from build123d import *

# Parameters (mm, degrees)
F0_W     = 122
F0_H     = 44
F0_R     = 2
F1_DEPTH = 1.6
F2_W     = 106
F2_H     = 35
F3_DEPTH = 8.5
F5_DEPTH = 3.5


with BuildPart() as f1:
    # F0 (on Front) → F1 (new body)
    with BuildSketch(Plane.XZ):
        Rectangle(F0_W, F0_H)
        with Locations((-57.5, -18.5)):
            Circle(F0_R, mode=Mode.SUBTRACT)
        with Locations((57.5, -18.5)):
            Circle(F0_R, mode=Mode.SUBTRACT)
        with Locations((-57.5, 18.5)):
            Circle(F0_R, mode=Mode.SUBTRACT)
        with Locations((57.5, 18.5)):
            Circle(F0_R, mode=Mode.SUBTRACT)
    extrude(amount=-F1_DEPTH)

    # F2 (on Front) → F3 (join)
    with BuildSketch(Plane.XZ):
        with Locations((0, 2.25)):
            Rectangle(F2_W, F2_H)
    extrude(amount=F3_DEPTH)

    # F4 (on Front) → F5 (join)
    with BuildSketch(Plane.XZ):
        Polygon((53, 15.300509), (53, -13.699491), (57.8, -8.899491), (57.8, 10.500509), align=None)
    extrude(amount=F5_DEPTH)


solid = f1.part
Geometry check sheet. Reference: the model listing, model coordinates, mm. A direction names the side the tool comes from. Round coordinates to 2 decimals unless told otherwise and drop trailing zeros. Order: outer loops, then holes, each group sorted by start corner. A loop starts at its lowest first (then second) coordinate and runs counter-clockwise, first axis right, second up. Notation, with made-up numbers: (16.5, 43) - (25.5, 43) arc R23 ccw to (25.5, 53) - close; hole circle Ø9 at (8, 19). An arc over 180 degrees is marked (long way). One line per question, with ' | ' between items. Start each with the question number.
(1) Sectioned sample at C-C on x = -57.5. Record the cut outline in (y, z).
(2) Access from +Z, -Z, +X, -X, +Y, -Y to the whole of each face (thin tool, end or side, straight path). Record for faces 1 (the flat face through (-53, -4, 2)), 2 (the flat face through (55.4, -1.7, 12.9)), 3 (the flat face through (57.8, -2, 1)), 4 (the flat face through (-1, -4, 19.75)), 5 (the flat face through (-1, -4, -15.25)).
(3) Thickness scan on L1, parallel to Z at x = -57.5, y = 0.3; L2, parallel to X at y = -0.5, z = 19; L3, parallel to Z at x = 11.5, y = -1. Record the ranges inside material, lowest first. Write a range as [from, to].
(4) Sectioned sample at D-D on x = -41. Record the cut outline in (y, z).
(5) Release check for a two-part mould opening along Z. For faces 6 (the flat face through (53, -6, 2)), 7 (the flat face through (55.4, -1.7, -11.3)), 8 (the cylindrical face through (59.408, 0.789, 19.101)) record: released by +Z, released by -Z, zero draft, split by the parting line, or undercut.
(6) Depth check by flat-ended pin: pin 1 Ø3 at (y, z) = (-2, 1.5) entering from +X; pin 2 Ø4 at (x, y) = (-33.5, -6.5) entering from +Z; pin 3 Ø1.5 at (x, y) = (-20.5, -5) entering from -Z. Enter the tip coordinate at first touch or a pass-through.
(7) Sectioned sample at B-B on y = -2. Record the cut outline in (x, z), and give its area (3 significant figures).
(8) Sectioned sample at A-A on z = -18.5. Record the cut outline in (x, y).
Conclusion:
1) outline: (0, -22) - (1.6, -22) - (1.6, -20.5) - (0, -20.5) - close; (0, -16.5) - (1.6, -16.5) - (1.6, 16.5) - (0, 16.5) - close; (0, 20.5) - (1.6, 20.5) - (1.6, 22) - (0, 22) - close
2) face 1: +Z, -Z, -X, -Y | face 2: +Z, +X, -Y | face 3: +Z, -Z, +X, -Y | face 4: +Z, +X, -X, -Y | face 5: -Z, +X, -X, -Y
3) L1: z = [-22, -20.5], [-16.5, 16.5], [20.5, 22] | L2: x = [-53, 53] | L3: z = [-15.25, 19.75]
4) outline: (-8.5, -15.25) - (0, -15.25) - (0, -22) - (1.6, -22) - (1.6, 22) - (0, 22) - (0, 19.75) - (-8.5, 19.75) - close
5) face 6: zero draft | face 7: released by -Z | face 8: undercut
6) pin 1: stops at x = 57.8 | pin 2: stops at z = 19.75 | pin 3: stops at z = -15.25
7) outline: (-53, -15.25) - (53, -15.25) - (53, -13.7) - (57.8, -8.9) - (57.8, 10.5) - (53, 15.3) - (53, 19.75) - (-53, 19.75) - close | area: 3,830 mm2
8) outline: (-61, 0) - (-59.5, 0) - (-59.5, 1.6) - (-61, 1.6) - close; (-55.5, 0) - (55.5, 0) - (55.5, 1.6) - (-55.5, 1.6) - close; (59.5, 0) - (61, 0) - (61, 1.6) - (59.5, 1.6) - close
